from build123d import *

# Parameters (mm, degrees)
CROQUIS1_R              = 49
SALIENTE_EXTRUIR1_DEPTH = 15
CROQUIS2_R              = 5
CORTAR_EXTRUIR1_DEPTH   = 71.901339903
CROQUIS3_R              = 25
CROQUIS3_R_2            = 13
SALIENTE_EXTRUIR2_DEPTH = 75
CROQUIS4_R              = 6
SALIENTE_EXTRUIR3_DEPTH = 15
CROQUIS5_R              = 17.5
CORTAR_EXTRUIR2_DEPTH   = 30


with BuildPart() as part:
    # Croquis1 → Saliente-Extruir1 (new body)
    with BuildSketch(Plane.XY):
        Circle(CROQUIS1_R)
    extrude(amount=SALIENTE_EXTRUIR1_DEPTH)

    # Croquis2 → Cortar-Extruir1 (cut, through all)
    with BuildSketch(Plane.XY.offset(15)):
        with Locations((0, 35)):
            Circle(CROQUIS2_R)
        with Locations((30.310889132, 17.5)):
            Circle(CROQUIS2_R)
        with Locations((30.310889132, -17.5)):
            Circle(CROQUIS2_R)
        with Locations((0, -35)):
            Circle(CROQUIS2_R)
        with Locations((-30.310889132, -17.5)):
            Circle(CROQUIS2_R)
        with Locations((-30.310889132, 17.5)):
            Circle(CROQUIS2_R)
    extrude(amount=-CORTAR_EXTRUIR1_DEPTH, mode=Mode.SUBTRACT)

    # Croquis3 → Saliente-Extruir2 (add)
    with BuildSketch(Plane.XY.offset(15)):
        Circle(CROQUIS3_R)
        Circle(CROQUIS3_R_2, mode=Mode.SUBTRACT)
    extrude(amount=SALIENTE_EXTRUIR2_DEPTH)

    # Croquis4 → Saliente-Extruir3 (add)
    with BuildSketch(Plane.XY.offset(90)):
        with BuildLine():
            Line((14.309088021, 54.5), (28.618176043, 9))
            ThreePointArc((28.618176043, 9), (30, 0), (28.618176043, -9))
            Line((28.618176043, -9), (14.309088021, -54.5))
            ThreePointArc((14.309088021, -54.5), (0, -65), (-14.309088021, -54.5))
            Line((-14.309088021, -54.5), (-28.618176043, -9))
            ThreePointArc((-28.618176043, -9), (-30, 0), (-28.618176043, 9))
            Line((-28.618176043, 9), (-14.309088021, 54.5))
            ThreePointArc((-14.309088021, 54.5), (0, 65), (14.309088021, 54.5))
        make_face()
        with Locations((0, 50)):
            Circle(CROQUIS4_R, mode=Mode.SUBTRACT)
        with Locations((0, -50)):
            Circle(CROQUIS4_R, mode=Mode.SUBTRACT)
    extrude(amount=-SALIENTE_EXTRUIR3_DEPTH)

    # Croquis5 → Cortar-Extruir2 (cut)
    with BuildSketch(Plane.XY.offset(90)):
        Circle(CROQUIS5_R)
    extrude(amount=-CORTAR_EXTRUIR2_DEPTH, mode=Mode.SUBTRACT)


solid = part.part
Input: part model. Units: mm. Frame: model coordinates. A direction names the side the tool comes from. Round coordinates to 2 decimals unless told otherwise and drop trailing zeros. Order: outer loops, then holes, each group sorted by start corner. A loop starts at its lowest first (then second) coordinate and runs counter-clockwise, first axis right, second up. Notation, with made-up numbers: (27, 43.25) - (82, 43.25) arc R22 ccw to (82, 79.25) - close; hole circle Ø4 at (50, -33.75). An arc over 180 degrees is marked (long way). Answer as a JSON object with one key per item and string values. Group by question number.
(1) Reachability of faces 4 (the face through (21.564, -31.432, 82.605)), 5 (the face through (-21.564, 31.432, 82.605)), 6 (the face through (-3, 13, 60)), 7 (the face through (-1.08, -39.88, 7.6)) from +Z, -Z, +X, -X, +Y, -Y: full face, straight path, thin tool, end or side. Return the list, or none.
(2) Draft query along X for faces 1 (the face through (0, 0, 15)), 2 (the face through (0, -65, 83)), 3 (the face through (21.363, 32.068, 82.605)). Return one class per face: released by +X, released by -X, zero draft, split by the parting line, or undercut.
(3) Cut plane B-B (y = 0). Return loops of the section in (x, z), then the cut area to 3 significant figures.
(4) Cut plane C-C (y = -15.5). Return loops of the section in (x, z), then the cut area to 3 significant figures.
(5) Cut plane A-A (z = 80). Return loops of the section in (x, y).
(6) Material intervals for probe 1 along Y at (x, z) = (0, 85); probe 2 along Z at (x, y) = (11, 32.5); probe 3 along Y at (x, z) = (0, 69), sorted ascending. Write a range as from..to.
(7) Pin query (flat end, axial travel): P1, Ø8, axis at x = 0, y = -3.5, coming from the +Z side; P2, Ø1.5, axis at x = -1, z = 11, coming from the +Y side; P3, Ø2, axis at x = -0.5, z = 31, coming from the -Y side. Return the tip coordinate at first contact, or that it passes through.
(8) Cut plane D-D (x = 0). Count the separate pieces of the cut face and the enclosed holes in it, then the cut area to 3 significant figures.
Here are the results:
{
 "1": {"face 4": "+Z, +X, -Y", "face 5": "+Z, -X, +Y", "face 6": "+Z", "face 7": "-Z"},
 "2": {"face 1": "undercut", "face 2": "split by the parting line", "face 3": "released by +X"},
 "3": {"outline": "(-49, 0) - (49, 0) - (49, 15) - (25, 15) - (25, 75) - (30, 75) - (30, 90) - (17.5, 90) - (17.5, 60) - (13, 60) - (13, 15) - (-13, 15) - (-13, 60) - (-17.5, 60) - (-17.5, 90) - (-30, 90) - (-30, 75) - (-25, 75) - (-25, 15) - (-49, 15) - close", "area": "3,150 mm^2"},
 "4": {"outline": "(-46.48, 0) - (-34.89, 0) - (-34.89, 15) - (-46.48, 15) - close; (-26.57, 75) - (-19.62, 75) - (-19.62, 15) - (-25.73, 15) - (-25.73, 0) - (25.73, 0) - (25.73, 15) - (19.62, 15) - (19.62, 75) - (26.57, 75) - (26.57, 90) - (8.12, 90) - (8.12, 60) - (-8.12, 60) - (-8.12, 90) - (-26.57, 90) - close; (34.89, 0) - (46.48, 0) - (46.48, 15) - (34.89, 15) - close", "area": "3,780 mm^2"},
 "5": {"outline": "(-28.62, -9) - (-14.31, -54.5) arc R15 ccw to (14.31, -54.5) - (28.62, -9) arc R30 ccw to (28.62, 9) - (14.31, 54.5) arc R15 ccw to (-14.31, 54.5) - (-28.62, 9) arc R30 ccw to start; hole circle Ø35 at (0, 0); hole circle Ø12 at (0, -50); hole circle Ø12 at (0, 50)"},
 "6": {"probe 1": "y = -65..-56, -44..-17.5, 17.5..44, 56..65", "probe 2": "z = 0..15, 75..90", "probe 3": "y = -25..-17.5, 17.5..25"},
 "7": {"P1": "stops at z = 15", "P2": "stops at y = 49", "P3": "stops at y = -25"},
 "8": {"separate pieces": "5", "enclosed holes": "0", "area": "3,540 mm^2"}
}
